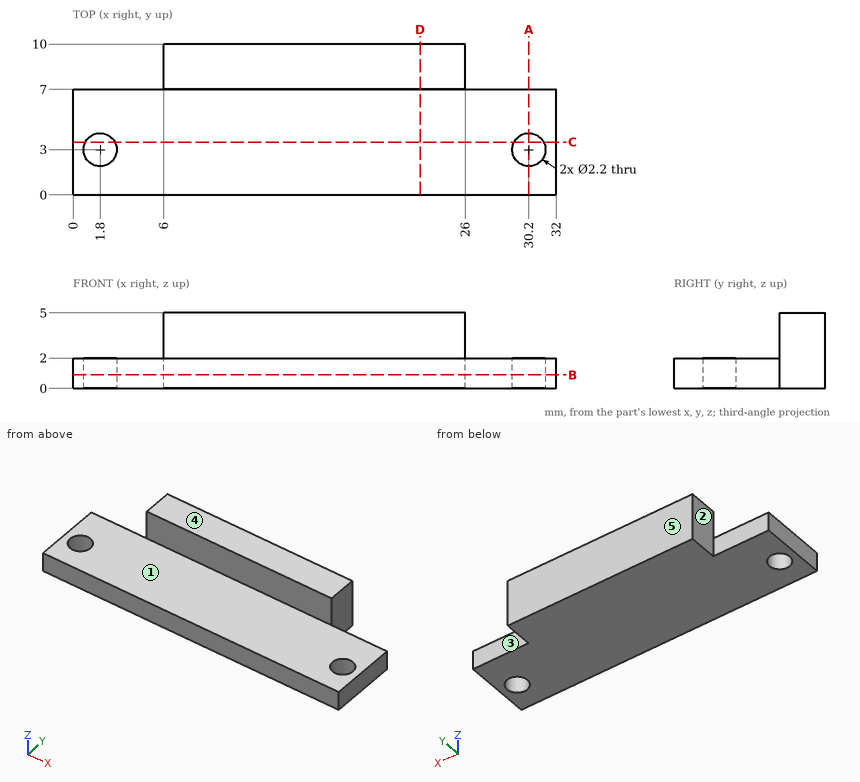
Input: dimensioned drawing with shaded views. Units: mm. Origin: part minimum x, y, z. A direction names the side the tool comes from. Give positions to 0.01 mm unless a question says otherwise; leave off trailing zeros. Write each loop counter-clockwise with the first axis right and the second up, starting at its lowest first coordinate (ties: lowest second). Pieces come first, ordered by that corner, then holes. Notation, with made-up numbers: (-25.5, -11.5) - (-19.5, -11.5) arc R23 cw to (-19.5, 23.5) - close; hole circle Ø11 at (38.25, 36.25). An arc over 180 degrees is marked (long way). Write item = value, one per line. Start each with the question number.
1) Cut plane A-A (x = 30.2). Return loops of the section in (y, z), and give its area (3 significant figures).
2) Reachability of the marked faces 1, 2, 3, 4 and 5 from +Z, -Z, +X, -X, +Y, -Y: full face, straight path, thin tool, end or side. Return the list, or none.
3) Pin query (flat end, axial travel): pin 1 (1 mm diameter, centred on y = 8, z = 1, fed in from -X); pin 2 (2 mm diameter, centred on x = 14.5, y = 4.5, fed in from +Z); pin 3 (0.6 mm diameter, centred on x = 2, z = 0.5, fed in from +Y); pin 4 (1.5 mm diameter, centred on y = 1, z = 3.5, fed in from +X). Return the tip coordinate at first contact, or that it passes through.
4) Material intervals for L1, parallel to Y at x = 1.8, z = 1.55; L2, parallel to Z at x = 9, y = 3.5; L3, parallel to Y at x = 19, z = 4.65, sorted ascending. Write a range as [from, to].
5) Cut plane B-B (z = 0.9). Return loops of the section in (x, y).
6) Cut plane C-C (y = 3.5). Return loops of the section in (x, z).
7) Cut plane D-D (x = 23). Return loops of the section in (y, z).
Answers follow:
q1.outline = (0, 0) - (1.9, 0) - (1.9, 2) - (0, 2) - close; (4.1, 0) - (7, 0) - (7, 2) - (4.1, 2) - close
q1.area = 9.60 mm^2
q2.face_1 = +Z, +X, -X, -Y
q2.face_2 = +Z, -Z, -X, +Y
q2.face_3 = +Z, -Z, +X, +Y
q2.face_4 = +Z, +X, -X, +Y, -Y
q2.face_5 = +Z, -Z, +X, -X, +Y
q3.pin_1 = 6
q3.pin_2 = 2
q3.pin_3 = 7
q3.pin_4 = through
q4.L1 = [0, 1.9], [4.1, 7]
q4.L2 = [0, 2]
q4.L3 = [7, 10]
q5.outline = (0, 0) - (32, 0) - (32, 7) - (26, 7) - (26, 10) - (6, 10) - (6, 7) - (0, 7) - close; hole circle Ø2.2 at (1.8, 3); hole circle Ø2.2 at (30.2, 3)
q6.outline = (0, 0) - (0.82, 0) - (0.82, 2) - (0, 2) - close; (2.78, 0) - (29.22, 0) - (29.22, 2) - (2.78, 2) - close; (31.18, 0) - (32, 0) - (32, 2) - (31.18, 2) - close
q7.outline = (0, 0) - (10, 0) - (10, 5) - (7, 5) - (7, 2) - (0, 2) - close
